Build history of the part. All positions in model axes, mm. Face numbers are marked on the shaded views. A direction names the side the tool comes from. Give positions to 0.01 mm unless a question says otherwise; leave off trailing zeros. Write each loop counter-clockwise with the first axis right and the second up, starting at its lowest first coordinate (ties: lowest second). Pieces come first, ordered by that corner, then holes. Notation, with made-up numbers: (-3.5, 13.5) -> (2.5, 13.5) arc R27 cw to (2.5, 51.5) -> close; hole circle Ø8 at (-34.75, -0.75). An arc over 180 degrees is marked (long way). One line per question, with ' | ' between items. Start each with the question number.
(1) Band-saw the part on B-B, the plane y = -16. Give the cut face in (x, z).
(2) Band-saw the part on A-A, the plane z = 6. Give the cut face in (x, y), and give its area (3 significant figures).
(3) Band-saw the part on D-D, the plane z = 36.5. Give the cut face in (x, y), and give its area (3 significant figures).
(4) Band-saw the part on C-C, the plane x = 0. Give the cut face in (y, z), and give its area (3 significant figures).
(5) Drill centre lines: probe 1 along Z at (x, y) = (-15, -28); probe 2 along Y at (x, z) = (0, 16); probe 3 along Y at (x, z) = (-0.5, 29). Where is each one in solid material? Low to high. Write a range as from..to.
(6) Pin check, flat tips, straight feed: P1, Ø8, axis at y = -8, z = 29.5, coming from the -X side; P2, Ø3, axis at x = 23.5, z = 5.5, coming from the -Y side; P3, Ø2, axis at x = 1, z = 37, coming from the -Y side. Stop position of each tip, or through.
(7) Tool access for the marked faces 1, 2 and 3: list every direction of +Z, -Z, +X, -X, +Y, -Y with a clear straight run to the whole face (end or side of a thin tool).
(8) Pull direction X, two halves, no side cores. Call the marked faces 4, 5 and 6: released by +X, released by -X, zero draft, split by the parting line, or undercut.
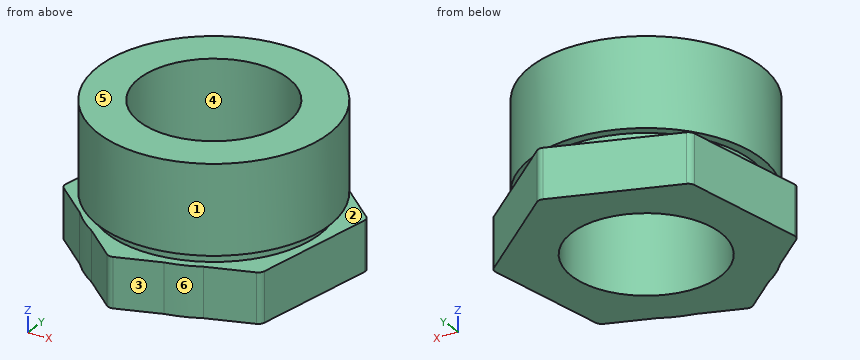
from build123d import *

# Parameters (mm, degrees)
SKETCH1_R           = 32.5
BOSS_EXTRUDE1_DEPTH = 42
CUT_EXTRUDE1_START  = -28
SKETCH2_R           = 32.5
SKETCH2_R_2         = 30
CUT_EXTRUDE1_DEPTH  = 3
BOSS_EXTRUDE2_DEPTH = 14
FILLET1_R           = 2
SKETCH4_R           = 21
CUT_EXTRUDE2_DEPTH  = 67.142933871


with BuildPart() as part:
    # Sketch1 → Boss-Extrude1 (new body)
    with BuildSketch(Plane.XY):
        with Locations(Location((0, 0, 0), (0, 0, 180))):
            Circle(SKETCH1_R)
    extrude(amount=BOSS_EXTRUDE1_DEPTH)

    # Sketch2 → Cut-Extrude1 (cut)
    with BuildSketch(Plane.XY.offset(42).offset(CUT_EXTRUDE1_START)):
        with Locations(Location((0, 0, 0), (0, 0, 180))):
            Circle(SKETCH2_R)
        Circle(SKETCH2_R_2, mode=Mode.SUBTRACT)
    extrude(amount=CUT_EXTRUDE1_DEPTH, mode=Mode.SUBTRACT)

    # Sketch3 → Boss-Extrude2 (add)
    with BuildSketch(Plane(origin=(0, 0, 0), x_dir=(-1, 0, 0), z_dir=(0, 0, -1))):
        Polygon((-35.269916777, 13.430130963), (-28.941400728, -23.560181525), (6.257407604, -36.574682103), (35.127699889, -12.598870193), (28.799183841, 24.391442295), (-6.399624492, 37.405942873), align=None)
    extrude(amount=-BOSS_EXTRUDE2_DEPTH)

    # Fillet1
    fillet1_edges = [part.edges().sort_by_distance(p)[0] for p in [
        (-28.799183841, 24.391442295, 7),
        (-35.127699889, -12.598870193, 7),
        (-6.257407604, -36.574682103, 7),
        (28.941400728, -23.560181525, 7),
        (35.269916777, 13.430130963, 7),
        (6.399624492, 37.405942873, 7),
    ]]
    fillet(fillet1_edges, radius=FILLET1_R)

    # Sketch4 → Cut-Extrude2 (cut, through all)
    with BuildSketch(Plane.XY.offset(42)):
        Circle(SKETCH4_R)
    extrude(amount=-CUT_EXTRUDE2_DEPTH, mode=Mode.SUBTRACT)


solid = part.part
Results:
1) outline: (-31.03, 0) -> (-13.6, 0) -> (-13.6, 42) -> (-28.29, 42) -> (-28.29, 17) -> (-25.38, 17) -> (-25.38, 14) -> (-31.03, 14) -> close; (13.6, 0) -> (30.23, 0) -> (30.23, 14) -> (25.38, 14) -> (25.38, 17) -> (28.29, 17) -> (28.29, 42) -> (13.6, 42) -> close
2) outline: (-34.93, -11.46) arc R2 ccw to (-34.24, -13.34) -> (-24.27, -21.62) arc R32.5 ccw to (-16.79, -27.83) -> (-7.15, -35.84) arc R2 ccw to (-5.17, -36.17) -> (6.59, -31.83) arc R32.5 ccw to (15.7, -28.46) -> (27.86, -23.96) arc R2 ccw to (29.14, -22.42) -> (35.08, 12.29) arc R2 ccw to (34.38, 14.17) -> (7.29, 36.67) arc R2 ccw to (5.32, 37.01) -> (-27.72, 24.79) arc R2 ccw to (-28.99, 23.25) -> close; hole circle Ø42 at (0, 0) | area: 2,280 mm²
3) outline: circle Ø65 at (0, 0); hole circle Ø42 at (0, 0) | area: 1,930 mm²
4) outline: (-34.26, 0) -> (-21, 0) -> (-21, 42) -> (-32.5, 42) -> (-32.5, 17) -> (-30, 17) -> (-30, 14) -> (-34.26, 14) -> close; (21, 0) -> (35.04, 0) -> (35.04, 14) -> (30, 14) -> (30, 17) -> (32.5, 17) -> (32.5, 42) -> (21, 42) -> close | area: 1,010 mm²
5) probe 1: z = 0..14, 17..42 | probe 2: y = -30..-21, 21..30 | probe 3: y = -32.5..-20.99, 20.99..32.5
6) P1: stops at x = -32.25 | P2: stops at y = -26.13 | P3: stops at y = -32.5
7) face 1: +Z | face 2: none | face 3: +Z, -Z, +X, -Y
8) face 4: undercut | face 5: zero draft | face 6: released by +X
